```python
from build123d import *

# Parameters (mm, degrees)
SKETCH1_R                 = 125
SKETCH1_R_2               = 45
SKETCH1_R_3               = 5
BOSS_EXTRUDE1_DEPTH       = 40
SKETCH3_R                 = 90
SKETCH3_R_2               = 72.5
BOSS_EXTRUDE2_DEPTH       = 14.5
CUT_EXTRUDE1_DEPTH        = 182.245689604
CUT_EXTRUDE1_DEPTH_BACK   = 182.245689604
SKETCH4_W                 = 14.5
SKETCH4_H                 = 90
SKETCH5_R                 = 100
CUT_EXTRUDE3_DEPTH        = 19.5
F_8_0MM_DOWEL_HOLE1_D     = 8
F_8_0MM_DOWEL_HOLE1_DEPTH = 10
F_8_0MM_DOWEL_HOLE1_TIP   = 2.403442476


with BuildPart() as part:
    # Sketch1 → Boss-Extrude1 (new body)
    with BuildSketch(Plane(origin=(0, 0, 0), x_dir=(0, 0, -1), z_dir=(1, 0, 0))):
        Circle(SKETCH1_R)
        Circle(SKETCH1_R_2, mode=Mode.SUBTRACT)
        with Locations((0, 107.5)):
            Circle(SKETCH1_R_3, mode=Mode.SUBTRACT)
        with Locations(Location((93.097730907, 53.75, 0), (0, 0, 180))):
            Circle(SKETCH1_R_3, mode=Mode.SUBTRACT)
        with Locations(Location((-93.097730907, 53.75, 0), (0, 0, 180))):
            Circle(SKETCH1_R_3, mode=Mode.SUBTRACT)
        with Locations((-93.097730907, -53.75)):
            Circle(SKETCH1_R_3, mode=Mode.SUBTRACT)
        with Locations(Location((0, -107.5, 0), (0, 0, 180))):
            Circle(SKETCH1_R_3, mode=Mode.SUBTRACT)
        with Locations((93.097730907, -53.75)):
            Circle(SKETCH1_R_3, mode=Mode.SUBTRACT)
    extrude(amount=-BOSS_EXTRUDE1_DEPTH)

    # Sketch3 → Boss-Extrude2 (add)
    with BuildSketch(Plane(origin=(0, 0, 0), x_dir=(0, 0, -1), z_dir=(1, 0, 0))):
        with Locations(Location((0, 0, 0), (0, 0, 180))):
            Circle(SKETCH3_R)
        with Locations(Location((0, 0, 0), (0, 0, 180))):
            Circle(SKETCH3_R_2, mode=Mode.SUBTRACT)
    extrude(amount=BOSS_EXTRUDE2_DEPTH)

    # Sketch4 → Cut-Extrude1 (cut, two sides: drawn at the far end of the back side and taken through both)
    with BuildSketch(Plane(origin=(0, 0, 0), x_dir=(1, 0, 0), z_dir=(0, 1, 0)).offset(-CUT_EXTRUDE1_DEPTH_BACK)):
        with Locations((7.25, 0)):
            Rectangle(SKETCH4_W, SKETCH4_H)
    extrude(amount=CUT_EXTRUDE1_DEPTH + CUT_EXTRUDE1_DEPTH_BACK, mode=Mode.SUBTRACT)

    # Sketch5 → Cut-Extrude3 (cut)
    with BuildSketch(Plane.ZY.offset(40)):
        Circle(SKETCH5_R)
    extrude(amount=-CUT_EXTRUDE3_DEPTH, mode=Mode.SUBTRACT)

    # Ø8.0mm Dowel Hole1
    with Locations(Plane.ZY.offset(20.5)):
        with Locations((0, 90), (77.942286341, 45), (77.942286341, -45), (0, -90), (-77.942286341, -45), (-77.942286341, 45)):
            Hole(F_8_0MM_DOWEL_HOLE1_D / 2, depth=F_8_0MM_DOWEL_HOLE1_DEPTH)
            with Locations((0, 0, -(F_8_0MM_DOWEL_HOLE1_DEPTH + F_8_0MM_DOWEL_HOLE1_TIP / 2))):  # 118° drill point
                Cone(0, F_8_0MM_DOWEL_HOLE1_D / 2, F_8_0MM_DOWEL_HOLE1_TIP, mode=Mode.SUBTRACT)


solid = part.part
```
Build history of the part. All positions in model axes, mm. A direction names the side the tool comes from. Give positions to 0.01 mm unless a question says otherwise; leave off trailing zeros. Loops run counter-clockwise (first coordinate to the right, second up) from the corner with the lowest first, then second, coordinate; pieces in that order, holes last. Notation, with made-up numbers: (87, 66) - (135, 66) arc R16 cw to (135, 86) - close; hole circle Ø7 at (5.5, 33). An arc over 180 degrees is marked (long way). Use a Markdown table: item, result.
(1) Band-saw the part on B-B (x = -33). Give the cut face in (y, z), and give its area (3 significant figures).
Taken from the geometry:
| item | result |
|---|---|
| outline | circle Ø250 at (0, 0); hole circle Ø10 at (-107.5, 0); hole circle Ø200 at (0, 0); hole circle Ø10 at (-53.75, -93.1); hole circle Ø10 at (-53.75, 93.1); hole circle Ø10 at (53.75, -93.1); hole circle Ø10 at (53.75, 93.1); hole circle Ø10 at (107.5, 0) |
| area | 17,200 mm2 |
(2) Band-saw the part on C-C (y = 16.5). Give the cut face in (x, z).
Taken from the geometry:
| item | result |
|---|---|
| outline | (-40, -123.91) - (0, -123.91) - (0, -88.47) - (14.5, -88.47) - (14.5, -70.6) - (0, -70.6) - (0, -41.87) - (-20.5, -41.87) - (-20.5, -98.63) - (-40, -98.63) - close; (-40, 98.63) - (-20.5, 98.63) - (-20.5, 41.87) - (0, 41.87) - (0, 70.6) - (14.5, 70.6) - (14.5, 88.47) - (0, 88.47) - (0, 123.91) - (-40, 123.91) - close |
(3) Pull direction Y, two halves, no side cores. Call faces 1 (the face through (-19.72, 102.62, 1.08)), 2 (the face through (7.15, 1.32, 89.99)), 3 (the face through (14.5, -1, 77)): +Y half, -Y half, draft (parallel to the pull), parting line (faces both ways), or undercut.
Taken from the geometry:
| item | result |
|---|---|
| face 1 | undercut |
| face 2 | parting line |
| face 3 | draft |
(4) Band-saw the part on D-D (z = 13). Give the cut face in (x, y), and give its area (3 significant figures).
Taken from the geometry:
| item | result |
|---|---|
| outline | (-40, -124.32) - (0, -124.32) - (0, -43.08) - (-20.5, -43.08) - (-20.5, -99.15) - (-40, -99.15) - close; (-40, 99.15) - (-20.5, 99.15) - (-20.5, 43.08) - (0, 43.08) - (0, 124.32) - (-40, 124.32) - close |
| area | 4,310 mm2 |
(5) Band-saw the part on A-A (x = 9). Give the cut face in (y, z).
Taken from the geometry:
| item | result |
|---|---|
| outline | (-77.94, -45) arc R90 ccw to (77.94, -45) - (56.84, -45) arc R72.5 cw to (-56.84, -45) - close; (-77.94, 45) - (-56.84, 45) arc R72.5 cw to (56.84, 45) - (77.94, 45) arc R90 ccw to start |
(6) Drop flat-ended pins along their axis: pin 1 Ø8 at (x, y) = (-21, -97.5) entering from -Z; pin 2 Ø13 at (y, z) = (107.5, 0) entering from +X; pin 3 Ø10 at (x, z) = (-34.5, -81.5) entering from -Y. Give the stop position or say it passes through.
Taken from the geometry:
| item | result |
|---|---|
| pin 1 | z = -82.96 |
| pin 2 | x = 0 |
| pin 3 | y = -98.86 |
(7) Which spindle directions (+Z, -Z, +X, -X, +Y, -Y) get a long thin tool onto all of the face, cutting with end or side? Do faces 4 (the face through (-19.72, 5.5, 124.88)), 5 (the face through (7.148, -0.915, -72.494)), 6 (the face through (-20.5, -43, 21)), 7 (the face through (7, -68, 45)), 8 (the face through (-40, -55, 84)). Say none if no direction does.
Taken from the geometry:
| item | result |
|---|---|
| face 4 | +X, -X |
| face 5 | +X |
| face 6 | -X |
| face 7 | +X, +Y, -Y |
| face 8 | +Z, -Z, -X, +Y, -Y |
(8) Wall check: line 1 along Y through (x, z) = (-14.25, 0); line 2 along Y through (x, z) = (-23, 0); line 3 along Y through (x, z) = (-15, -1). Give the ranges that are in metal, low to high.
Taken from the geometry:
| item | result |
|---|---|
| line 1 | -125 to -112.5, -102.5 to -94, -86 to -45, 45 to 86, 94 to 102.5, 112.5 to 125 |
| line 2 | -125 to -112.5, -102.5 to -100, 100 to 102.5, 112.5 to 125 |
| line 3 | -125 to -112.4, -102.6 to -93.87, -86.13 to -44.99, 44.99 to 86.13, 93.87 to 102.6, 112.4 to 125 |
